Here's how the part is built. I have some questions about the finished solid (model axes, mm). Give positions to 0.01 mm unless a question says otherwise; leave off trailing zeros. Write each loop counter-clockwise with the first axis right and the second up, starting at its lowest first coordinate (ties: lowest second). Pieces come first, ordered by that corner, then holes. Notation, with made-up numbers: M 34,86.5 L 54,86.5 A19 ccw 54,106.5 Z; hole C 33.25,-40 d10. An arc over 180 degrees is marked long. Answer as CSV lines item,"result". Start each with the question number.
Q1. Suppose I cut it at A-A (z = 56). Write out the boundary of the cut face in (x, y), then the cut area to 3 significant figures.
Q2. For pin 1 (1.5 mm diameter, centred on y = -2, z = 66, fed in from -X); pin 2 (1.5 mm diameter, centred on y = -1.5, z = 15.5, fed in from +X); pin 3 (2 mm diameter, centred on y = -1.5, z = 48, fed in from -X), each with a flat end and sliding along its axis, tell me the tip position at first contact or that it passes through.
Q3. Suppose I cut it at B-B (y = 0). Write out the boundary of the cut face in (x, z).
Q4. Suppose I cut it at C-C (z = 75). Write out the boundary of the cut face in (x, y).
Q5. If I drill on line 1 along Y through (x, z) = (-0.2, 80); line 2 along X through (y, z) = (1.1, 80) (3 decimals); line 3 along X through (y, z) = (1.35, 76), over which ranges is the centre line in solid material (lowest first)?
```python
from build123d import *

# Parameters (mm, degrees)
SKETCH1_R               = 2.5
EXTRUDE1_DEPTH          = 84
FILLET1_R               = 0.25
CUT_EXTRUDE1_DEPTH      = 3
CUT_EXTRUDE1_DEPTH_BACK = 3


with BuildPart() as part:
    # Sketch1 → Extrude1 (new body)
    with BuildSketch(Plane.XY):
        Circle(SKETCH1_R)
    extrude(amount=EXTRUDE1_DEPTH)

    # Fillet1
    fillet1_edges = [part.edges().sort_by_distance(p)[0] for p in [
        (-2.5, 0, 84),
    ]]
    fillet(fillet1_edges, radius=FILLET1_R)

    # Sketch2 → Cut-Extrude1 (cut, two sides)
    with BuildSketch(Plane(origin=(0, 0, 0), x_dir=(1, 0, 0), z_dir=(0, 1, 0))) as cut_extrude1_sk:
        with BuildLine():
            Line((-1.4, -84), (-1.4, -69))
            ThreePointArc((-1.4, -69), (-1.806967498, -68.194821478), (-2.696624903, -68.045005934))
            Line((-2.696624903, -68.045005934), (-2.696624903, -84))
            Line((-2.696624903, -84), (-1.4, -84))
        make_face()
    extrude(amount=CUT_EXTRUDE1_DEPTH, mode=Mode.SUBTRACT)
    extrude(cut_extrude1_sk.sketch, amount=-CUT_EXTRUDE1_DEPTH_BACK, mode=Mode.SUBTRACT)


solid = part.part
```
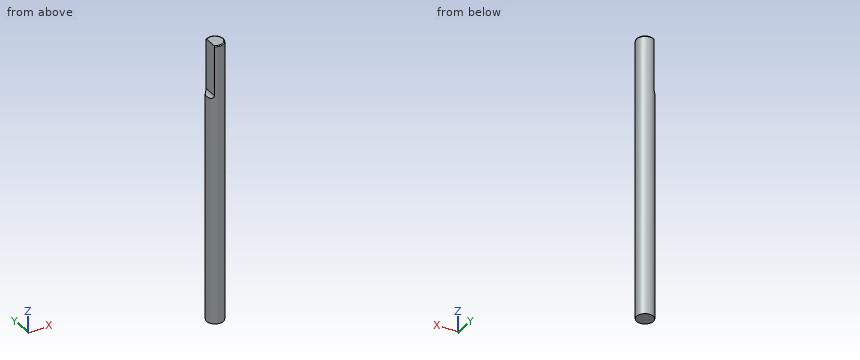
Resolved:
1,outline,"C 0,0 d5"
1,area,"19.6 mm^2"
2,pin 1,"x = -2.17"
2,pin 2,"x = 2.38"
2,pin 3,"x = -2.45"
3,outline,"M -2.5,0 L 2.5,0 L 2.5,83.75 A0.25 ccw 2.25,84 L -1.4,84 L -1.4,69 A1 cw -2.5,68.01 Z"
4,outline,"M -1.4,-2.07 A2.5 ccw long -1.4,2.07 Z"
5,line 1,"-2.49 to 2.49"
5,line 2,"-1.4 to 2.245"
5,line 3,"-1.4 to 2.1"
